Study the drawing (mm; zero at the part's minimum x, y, z) and answer. A direction names the side the tool comes from. Round coordinates to 2 decimals unless told otherwise and drop trailing zeros. Order: outer loops, then holes, each group sorted by start corner. A loop starts at its lowest first (then second) coordinate and runs counter-clockwise, first axis right, second up. Notation, with made-up numbers: (4.5, 62) - (17.5, 62) arc R28 cw to (17.5, 91) - close; hole circle Ø3 at (67.25, 8.25). An arc over 180 degrees is marked (long way). Use one line per item in the form item = value. Start each with the question number.
Q1. Find the intervals of material crossed by line 1 (X direction, y = 17, z = 2.1); line 2 (Y direction, x = 9.5, z = 1); line 3 (Y direction, x = 6.25, z = 1.6), in increasing order. Write a range as [from, to].
Q2. Which of the six approach directions +Z, -Z, +X, -X, +Y, -Y give full straight-line access (tool end or side, diameter ignored) to the marked faces 1, 2 and 3?
Q3. The part is cut by section A-A on y = 14. Determine the outline of the cut face in (x, z).
Q4. Given P1, Ø5, axis at x = 11.5, y = 9.5, coming from the -Z side; P2, Ø2.5, axis at x = 10.5, z = 2, coming from the -Y side; P3, Ø2, axis at x = 6, z = 1.5, coming from the -Y side, each flat-ended and moving along its own axis, determine where each tip first touches the part or whether it passes through.
Q5. For a pull along X with two mould halves and no side action, classify the marked faces 4, 5, 6 and 7 as +X half, -X half, draft (parallel to the pull), parting line (faces both ways), or undercut.
Q6. The part is cut by section B-B on z = 4.9. Determine the outline of the cut face in (x, y), plus the area to 3 significant figures.
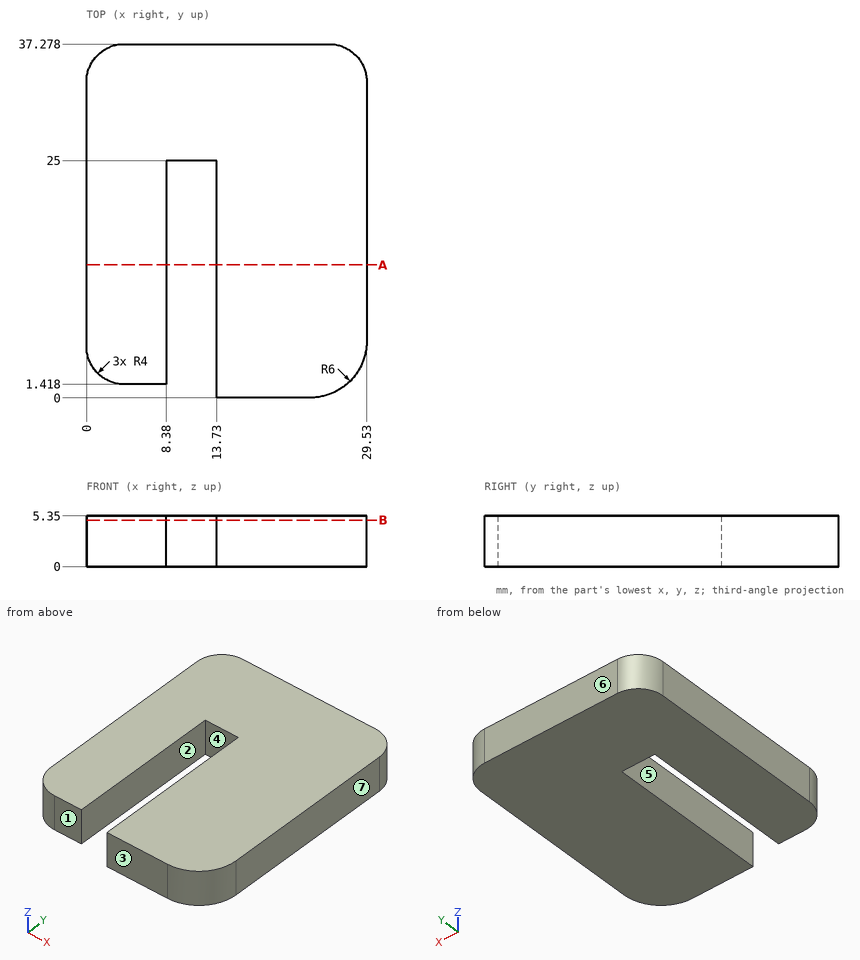
Found:
q1.line_1 = [0, 8.38], [13.73, 29.53]
q1.line_2 = [25, 37.28]
q1.line_3 = [1.42, 37.28]
q2.face_1 = +Z, -Z, -X, -Y
q2.face_2 = +Z, -Z, -Y
q2.face_3 = +Z, -Z, +X, -X, -Y
q3.outline = (0, 0) - (8.38, 0) - (8.38, 5.35) - (0, 5.35) - close; (13.73, 0) - (29.53, 0) - (29.53, 5.35) - (13.73, 5.35) - close
q4.P1 = 0
q4.P2 = 25
q4.P3 = 1.42
q5.face_4 = undercut
q5.face_5 = undercut
q5.face_6 = draft
q5.face_7 = +X half
q6.outline = (0, 5.42) arc R4 ccw to (4, 1.42) - (8.38, 1.42) - (8.38, 25) - (13.73, 25) - (13.73, 0) - (23.53, 0) arc R6 ccw to (29.53, 6) - (29.53, 33.28) arc R4 ccw to (25.53, 37.28) - (4, 37.28) arc R4 ccw to (0, 33.28) - close
q6.area = 937 mm²
